```python
from build123d import *

# Parameters (mm, degrees)
ESQUISSE1_R                  = 3
BOSS_EXTRU_1_DEPTH           = 28.5
ENL_V_MAT_EXTRU_1_DEPTH      = 29.814059068
ENL_V_MAT_EXTRU_1_DEPTH_BACK = 29.814059068
ESQUISSE2_R                  = 1.5
CHANFREIN1_SIZE              = 1


with BuildPart() as part:
    # Esquisse1 → Boss.-Extru.1 (new body)
    with BuildSketch(Plane.XY):
        with Locations(Location((0, 0, 0), (0, 0, 180))):
            Circle(ESQUISSE1_R)
    extrude(amount=BOSS_EXTRU_1_DEPTH)

    # Esquisse2 → Enlèv. mat.-Extru.1 (cut, two sides: drawn at the far end of the back side and taken through both)
    with BuildSketch(Plane(origin=(0, 0, 0), x_dir=(1, 0, 0), z_dir=(0, 1, 0)).offset(-ENL_V_MAT_EXTRU_1_DEPTH_BACK)):
        with Locations(Location((0, -3, 0), (0, 0, 270))):
            Circle(ESQUISSE2_R)
    extrude(amount=ENL_V_MAT_EXTRU_1_DEPTH + ENL_V_MAT_EXTRU_1_DEPTH_BACK, mode=Mode.SUBTRACT)

    # Chanfrein1
    chanfrein1_edges = [part.edges().sort_by_distance(p)[0] for p in [
        (3, 0, 28.5),
    ]]
    chamfer(chanfrein1_edges, length=CHANFREIN1_SIZE)


solid = part.part
```
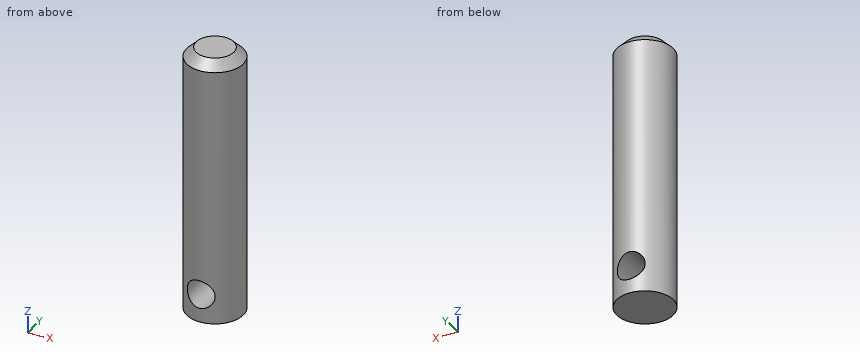
Input: part model. Units: mm. Frame: model coordinates. Coordinates: 2 decimals unless noted, no trailing zeros. Loops run counter-clockwise (first coordinate to the right, second up) from the corner with the lowest first, then second, coordinate; pieces in that order, holes last.
Q1. Section C-C, the plane z = 7.75. Return the cut outline in (x, y).
Results are:
outline: circle Ø6 at (0, 0)
Q2. Section A-A, the plane x = 0. Return the cut outline in (y, z), and give its area (3 significant figures).
Results are:
outline: (-3, 0) - (3, 0) - (3, 1.5) - (-3, 1.5) - close; (-3, 4.5) - (3, 4.5) - (3, 27.5) - (2, 28.5) - (-2, 28.5) - (-3, 27.5) - close
area: 152 mm2
Q3. Section B-B, the plane y = 0. Return the cut outline in (x, z).
Results are:
outline: (-3, 0) - (3, 0) - (3, 27.5) - (2, 28.5) - (-2, 28.5) - (-3, 27.5) - close; hole circle Ø3 at (0, 3)
Q4. Line query: line 1 along Z through (x, y) = (0, 1.5); line 2 along X through (y, z) = (1.5, 3); line 3 along X through (y, z) = (-1, 3). Output: solid intervals per line, ascending.
Results are:
line 1: z = 0 to 1.5, 4.5 to 28.5
line 2: x = -2.6 to -1.5, 1.5 to 2.6
line 3: x = -2.83 to -1.5, 1.5 to 2.83
Q5. Contact query for a flat-ended pin moving along its axis: pin 1 (1.5 mm diameter, centred on x = -2.5, z = 4.5, fed in from -Y). Output: stop coordinate, or through.
Results are:
pin 1: stops at y = -2.44
Q6. Section D-D, the plane z = 2. Return the cut outline in (x, y).
Results are:
outline: (-1.12, -2.78) - (-1.12, 2.78) arc R3 ccw to start; (1.12, -2.78) arc R3 ccw to (1.12, 2.78) - close
